```python
from build123d import *

# Parameters (mm, degrees)
F0_R            = 10
F0_R_2          = 6.1
F1_DEPTH        = 7
F3_DEPTH        = 7
F3_COPIES_COUNT = 8
F4_W            = 0.8
F4_H            = 2
F5_DEPTH        = 0.6
F6_T1_DEPTH     = 3.25


# Not quite as in the source:
# - a fillet or chamfer that OpenCascade refuses, or shapes differently, is made with other operations: its cross-section is extruded or revolved along the edge and cut away or added
# - a pattern or mirror of a feature is missing from the dataset's text; its kind, count and spacing are read off the source's solid


with BuildPart() as f1:
    # F0 (on Front) → F1 (new body)
    with BuildSketch(Plane.XZ):
        with Locations((0, -1.9)):
            Circle(F0_R)
        Circle(F0_R_2, mode=Mode.SUBTRACT)
    extrude(amount=F1_DEPTH)

    # F2 (on face) → F3 (cut)
    with BuildSketch(Plane.XZ.offset(7)):
        with BuildLine():
            Line((6.9913417162, 0.4619397663), (6.0396188995, 0.8561562646))
            ThreePointArc((6.0396188995, 0.8561562646), (6.0848860008, 0.429141418), (6.1, 0))
            ThreePointArc((6.1, 0), (6.0848860008, -0.429141418), (6.0396188995, -0.8561562646))
            Line((6.0396188995, -0.8561562646), (6.9913417162, -0.4619397663))
            ThreePointArc((6.9913417162, -0.4619397663), (7.3, 0), (6.9913417162, 0.4619397663))
        make_face()
    f3 = extrude(amount=-F3_DEPTH, mode=Mode.SUBTRACT)

    # F3_copies: F3 ×8 about axis
    f3_copies_axis = Axis((0, 0, 0), (0, 1, 0))
    for i in range(1, F3_COPIES_COUNT):
        add(f3.rotate(f3_copies_axis, i * 360 / F3_COPIES_COUNT), mode=Mode.SUBTRACT)

    # F4 (on face) → F5 (cut)
    with BuildSketch(Plane(origin=(0, 0, 0), x_dir=(-1, 0, 0), z_dir=(0, 1, 0))):
        with Locations((0, -9.3)):
            Rectangle(F4_W, F4_H)
    extrude(amount=-F5_DEPTH, mode=Mode.SUBTRACT)

    # F6: fillet of radius 0.5 on 2 edges, made by hand

    # F6_s2 → F6_t1 (join)
    with BuildSketch(Plane.XY.offset(-11.55)):
        with BuildLine():
            ThreePointArc((0.4, -0.1), (0.2535533906, -0.4535533906), (-0.1, -0.6))
            Line((-0.1, -0.6), (0.4, -0.6))
            Line((0.4, -0.6), (0.4, -0.1))
        make_face()
        with BuildLine():
            ThreePointArc((-0.4, -0.1), (-0.2535533906, -0.4535533906), (0.1, -0.6))
            Line((0.1, -0.6), (-0.4, -0.6))
            Line((-0.4, -0.6), (-0.4, -0.1))
        make_face()
    extrude(amount=F6_T1_DEPTH)


solid = f1.part
```
Geometry: final body of the model. Coordinates: model frame, mm. Round coordinates to 2 decimals unless told otherwise and drop trailing zeros. Loops run counter-clockwise (first coordinate to the right, second up) from the corner with the lowest first, then second, coordinate; pieces in that order, holes last.
Item 1: Contact query for flat-ended pins moving along their axis: P1, Ø2, axis at x = -4.5, y = -2.5, coming from the -Z side; P2, Ø2, axis at y = -5, z = 4.5, coming from the +X side; P3, Ø2, axis at x = -0.5, z = 3.5, coming from the -Y side; P4, Ø1.5, axis at y = -3.5, z = 6, coming from the +X side. Output: stop coordinate, or through.
Checked values:
P1: stops at z = -11.27
P2: stops at x = 8.42
P3: passes through
P4: stops at x = 6.99
Item 2: Section D-D, the plane x = -8. Output: boundary loops of the cut face in (y, z).
Checked values:
outline: (-7, -7.9) - (0, -7.9) - (0, 4.1) - (-7, 4.1) - close
Item 3: Line query: L1, parallel to X at y = -5.75, z = 5.25; L2, parallel to X at y = -6.5, z = -5.25; L3, parallel to Z at x = -5, y = -4.75. Output: solid intervals per line, ascending.
Checked values:
L1: x = -6.99 to -5.04, -4.57 to -3.11, 3.11 to 4.57, 5.04 to 6.99
L2: x = -9.42 to -5.04, -4.57 to -3.11, 3.11 to 4.57, 5.04 to 9.42
L3: z = -10.56 to -5.27, -3.96 to -3.49, 3.49 to 3.96, 5.27 to 6.76
Item 4: Section C-C, the plane z = -1.9. Output: boundary loops of the cut face in (x, y).
Checked values:
outline: (-10, -7) - (-5.8, -7) - (-5.8, 0) - (-10, 0) - close; (5.8, -7) - (10, -7) - (10, 0) - (5.8, 0) - close
Item 5: Mould query, pull axis X, two halves, no side actions, for faces 1 (the flat face through (2, -7, -6)), 2 (the flat face through (-6.51, -3.55, 0.66)). Classes: released by +X, released by -X, zero draft, split by the parting line, or undercut.
Checked values:
face 1: zero draft
face 2: undercut
Item 6: Section B-B, the plane z = 2.5. Output: boundary loops of the cut face in (x, y).
Checked values:
outline: (-8.98, -7) - (-5.56, -7) - (-5.56, 0) - (-8.98, 0) - close; (5.56, -7) - (8.98, -7) - (8.98, 0) - (5.56, 0) - close
